The model under review builds one solid part; all positions refer to its coordinate system, in mm. A direction names the side the tool comes from. Round coordinates to 2 decimals unless told otherwise and drop trailing zeros. Write each loop counter-clockwise with the first axis right and the second up, starting at its lowest first coordinate (ties: lowest second). Pieces come first, ordered by that corner, then holes. Notation, with made-up numbers: (69.25, 57.25) - (128.25, 57.25) arc R30 ccw to (128.25, 86.25) - close; hole circle Ø10 at (68, 77.5). An arc over 180 degrees is marked (long way). Use one line per item in the form item = value.
from build123d import *

# Parameters (mm, degrees)
SKETCH1_W           = 56.9849
SKETCH1_H           = 4.191
BOSS_EXTRUDE2_DEPTH = 10.07745
CUT_EXTRUDE2_DEPTH  = 6.223
FILLET8_R           = 6.223
CUT_EXTRUDE5_DEPTH  = 37.991848321


with BuildPart() as part:
    # Sketch1 → Boss-Extrude2 (new, symmetric)
    with BuildSketch(Plane(origin=(0, 0, 0), x_dir=(1, 0, 0), z_dir=(0, 1, 0))):
        with Locations((2.101827362, 14.315884605)):
            Rectangle(SKETCH1_W, SKETCH1_H)
        with BuildLine():
            Line((-26.390622638, 12.220384605), (5.236321347, -1.174073262))
            ThreePointArc((5.236321347, -1.174073262), (9.008282942, -1.735261042), (12.579803169, -0.398522749))
            Line((12.579803169, -0.398522749), (30.594277362, 12.220384605))
            Line((30.594277362, 12.220384605), (-26.390622638, 12.220384605))
        make_face()
    extrude(amount=BOSS_EXTRUDE2_DEPTH, both=True)

    # Sketch1<16> → Cut-Extrude2 (cut, symmetric)
    with BuildSketch(Plane(origin=(0, 0, 0), x_dir=(1, 0, 0), z_dir=(0, 1, 0))):
        with BuildLine():
            Line((-26.390622638, 12.220384605), (5.236321347, -1.174073262))
            ThreePointArc((5.236321347, -1.174073262), (9.008282942, -1.735261042), (12.579803169, -0.398522749))
            Line((12.579803169, -0.398522749), (30.594277362, 12.220384605))
            Line((30.594277362, 12.220384605), (-26.390622638, 12.220384605))
        make_face()
    extrude(amount=CUT_EXTRUDE2_DEPTH, both=True, mode=Mode.SUBTRACT)

    # Fillet8
    fillet8_edges = [part.edges().sort_by_distance(p)[0] for p in [
        (2.101827362, 6.223, -12.220384605),
        (2.101827362, -6.223, -12.220384605),
    ]]
    fillet(fillet8_edges, radius=FILLET8_R - 0.0001)  # a hair under: the kernel refuses the full size

    # Sketch3 → Cut-Extrude5 (cut, through all)
    with BuildSketch(Plane(origin=(0, 0, -16.411384605), x_dir=(-1, 0, 0), z_dir=(0, 0, -1))):
        with BuildLine():
            Line((-12.211027362, -6.223), (8.007372638, -6.223))
            ThreePointArc((8.007372638, -6.223), (9.803423862, -5.479051224), (10.547372638, -3.683))
            Line((10.547372638, -3.683), (10.547372638, 3.683))
            ThreePointArc((10.547372638, 3.683), (9.803423862, 5.479051224), (8.007372638, 6.223))
            Line((8.007372638, 6.223), (-12.211027362, 6.223))
            ThreePointArc((-12.211027362, 6.223), (-14.007078586, 5.479051224), (-14.751027362, 3.683))
            Line((-14.751027362, 3.683), (-14.751027362, -3.683))
            ThreePointArc((-14.751027362, -3.683), (-14.007078586, -5.479051224), (-12.211027362, -6.223))
        make_face()
    extrude(amount=-CUT_EXTRUDE5_DEPTH, mode=Mode.SUBTRACT)


solid = part.part
(1) Add section D-D on x = 10. Write out the cut boundary in (y, z).
Geometry results:
outline = (-10.08, -16.41) - (-6.22, -16.41) - (-6.22, 1.56) - (-10.08, 1.56) - close; (6.22, -16.41) - (10.08, -16.41) - (10.08, 1.56) - (6.22, 1.56) - close
(2) Machinability: for faces 4 (the flat face through (2, -10.077, -9)), 5 (the cylindrical face through (13.69, -5.75, -12.43)), 6 (the cylindrical face through (-17.328, -3.513, -11.134)), which of the approach directions +Z, -Z, +X, -X, +Y, -Y give a long, thin tool a straight path to every point of the face, cutting with its end or side? Answer none if there is none.
Geometry results:
face_4 = +Z, -Z, +X, -X, -Y
face_5 = +Z, -Z
face_6 = +Z, +X, -X
(3) Add section A-A on z = -13.5. Write out the cut boundary in (x, y).
Geometry results:
outline = (-26.39, -10.08) - (30.59, -10.08) - (30.59, 10.08) - (-26.39, 10.08) - close; hole (-10.55, -3.68) arc R2.54 ccw to (-8.01, -6.22) - (12.21, -6.22) arc R2.54 ccw to (14.75, -3.68) - (14.75, 3.68) arc R2.54 ccw to (12.21, 6.22) - (-8.01, 6.22) arc R2.54 ccw to (-10.55, 3.68) - close
(4) Insertion check: P1, Ø1, axis at x = -9, y = 5, coming from the +Z side; P2, Ø8, axis at x = -16.5, y = -7, coming from the +Z side; P3, Ø8, axis at x = 18.5, y = -5, coming from the +Z side. Each pin has a flat end and moves straight along its axis. Give the tip position at first contact, or say it passes through.
Geometry results:
P1 = through
P2 = -6.34
P3 = -1.08
(5) Add section B-B on y = -2.5. Write out the cut boundary in (x, z), then the cut area to 3 significant figures.
Geometry results:
outline = (-26.39, -16.41) - (-10.55, -16.41) - (-10.55, -11.7) - (-25.15, -11.7) - (-26.39, -12.22) - close; (14.75, -16.41) - (30.59, -16.41) - (30.59, -12.22) - (29.85, -11.7) - (14.75, -11.7) - close
area = 149 mm2
(6) Add section C-C on z = -8.25. Write out the cut boundary in (x, y).
Geometry results:
outline = (-17.02, -10.08) - (24.93, -10.08) - (24.93, -5.8) - (13.61, -5.8) arc R2.54 cw to (12.21, -6.22) - (-8.01, -6.22) arc R2.54 cw to (-9.41, -5.8) - (-17.02, -5.8) - close; (-17.02, 5.8) - (-9.41, 5.8) arc R2.54 cw to (-8.01, 6.22) - (12.21, 6.22) arc R2.54 cw to (13.61, 5.8) - (24.93, 5.8) - (24.93, 10.08) - (-17.02, 10.08) - close
(7) The part is to be moulded in two halves that separate along X. For faces 1 (the flat face through (23.463, -8.327, -7.225)), 2 (the cylindrical face through (-9.487, 5.748, -12.434)), 3 (the flat face through (-10.799, 7.349, -5.617)), say which applies: +X half, -X half, draft (parallel to the pull), parting line (faces both ways), or undercut.
Geometry results:
face_1 = +X half
face_2 = undercut
face_3 = -X half
(8) To check wall thickness, follow L1, parallel to X at y = -1.5, z = -12.25; L2, parallel to Y at x = 10.5, z = -10.75; L3, parallel to Y at x = 21, z = -8.25. State the ranges of each line that lie inside material, in increasing order.
Geometry results:
L1 = -26.39 to -10.55, 14.75 to 30.59
L2 = -10.08 to -6.22, 6.22 to 10.08
L3 = -10.08 to -5.8, 5.8 to 10.08
